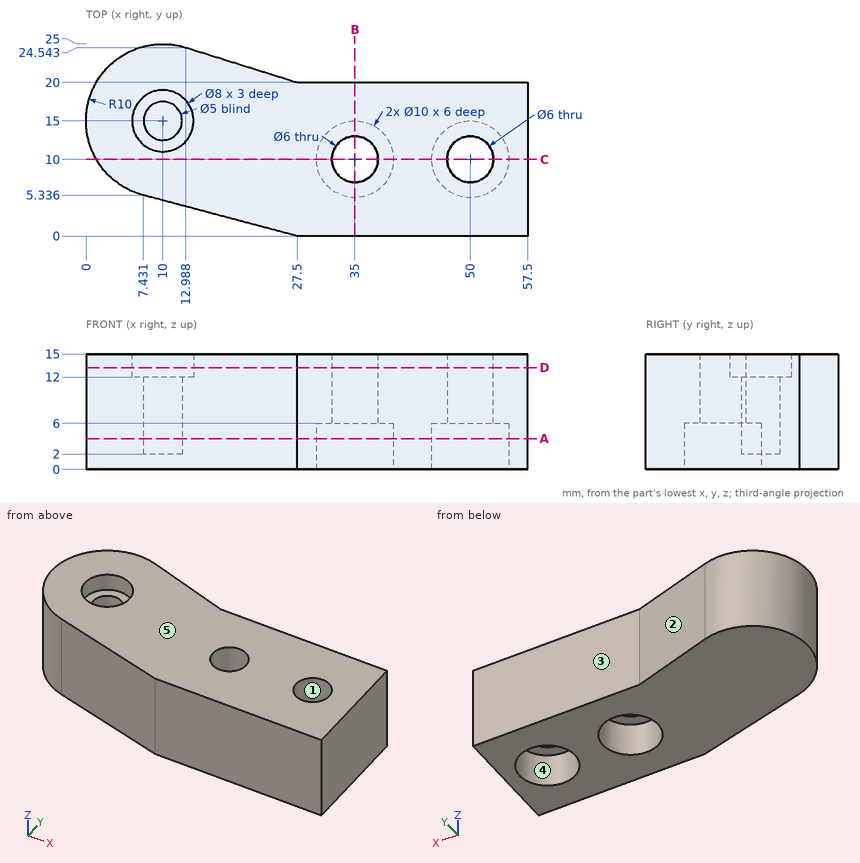
Design review of the part shown in the three views and the two pictorial views. Dimensions are in mm from the part's minimum x, y and z. A direction names the side the tool comes from. Round coordinates to 2 decimals unless told otherwise and drop trailing zeros. Loops run counter-clockwise (first coordinate to the right, second up) from the corner with the lowest first, then second, coordinate; pieces in that order, holes last.
(1) Wall thickness on line 1 along Y through (x, z) = (50, 2.4); line 2 along Z through (x, y) = (10, 16); line 3 along Y through (x, z) = (10, 13.2): over which ranges is each line inside the solid? List them lowest first.
Returned:
line 1: y = 0 to 5, 15 to 20
line 2: z = 0 to 2
line 3: y = 4.65 to 11, 19 to 25
(2) We need section B-B (x = 35). Give the boundary of the cut face in (y, z).
Returned:
outline: (0, 0) - (5, 0) - (5, 6) - (7, 6) - (7, 15) - (0, 15) - close; (13, 6) - (15, 6) - (15, 0) - (20, 0) - (20, 15) - (13, 15) - close
(3) Mouldability with a two-part tool opening along X and no side actions: class the marked faces 1, 2 and 3 as released by +X, released by -X, zero draft, split by the parting line, or undercut.
Returned:
face 1: undercut
face 2: released by +X
face 3: zero draft
(4) Clearance check with flat-ended pins moving along their axes: P1, Ø4, axis at x = 10, y = 13.5, coming from the +Z side; P2, Ø2, axis at x = 29, z = 13, coming from the +Y side; P3, Ø1.5, axis at x = 9.5, y = 14, coming from the +Z side. State where each tip first meets the part, or that it passes through.
Returned:
P1: stops at z = 12
P2: stops at y = 20
P3: stops at z = 2
(5) We need section D-D (z = 13.25). Give the boundary of the cut face in (x, y) (1 decimal), plus the area to 3 significant figures.
Returned:
outline: (7.4, 5.3) - (27.5, 0) - (57.5, 0) - (57.5, 20) - (27.5, 20) - (13, 24.5) arc R10 ccw (long way) to start; hole circle Ø8 at (10, 15); hole circle Ø6 at (35, 10); hole circle Ø6 at (50, 10)
area: 1,010 mm2
(6) We need section A-A (z = 4). Give the boundary of the cut face in (x, y) (1 decimal).
Returned:
outline: (7.4, 5.3) - (27.5, 0) - (57.5, 0) - (57.5, 20) - (27.5, 20) - (13, 24.5) arc R10 ccw (long way) to start; hole circle Ø5 at (10, 15); hole circle Ø10 at (35, 10); hole circle Ø10 at (50, 10)
(7) Tool access review of the marked faces 4 and 5: name each direction out of +Z, -Z, +X, -X, +Y, -Y from which nothing blocks a thin tool from reaching the whole face with its end or side.
Returned:
face 4: -Z
face 5: +Z, +X, -X, +Y, -Y
(8) We need section C-C (y = 10). Give the boundary of the cut face in (x, z).
Returned:
outline: (1.34, 0) - (30, 0) - (30, 6) - (32, 6) - (32, 15) - (1.34, 15) - close; (38, 6) - (40, 6) - (40, 0) - (45, 0) - (45, 6) - (47, 6) - (47, 15) - (38, 15) - close; (53, 6) - (55, 6) - (55, 0) - (57.5, 0) - (57.5, 15) - (53, 15) - close
